CAD build for the part. Positions are in the model's coordinates, mm. A direction names the side the tool comes from. Give positions to 0.01 mm unless a question says otherwise; leave off trailing zeros. Loops run counter-clockwise (first coordinate to the right, second up) from the corner with the lowest first, then second, coordinate; pieces in that order, holes last. Notation, with made-up numbers: (26.25, 15.5) - (43.25, 15.5) arc R18 cw to (43.25, 35.5) - close; hole circle Ø4 at (-4, 28). An arc over 180 degrees is marked (long way). Return JSON: item names as keys, results as strings.
from build123d import *

# Parameters (mm, degrees)
F0_W     = 970
F0_H     = 1730
F1_DEPTH = 50
F3_DEPTH = 50


with BuildPart() as f1:
    # F0 (on Front) → F1 (new body)
    with BuildSketch(Plane.XZ):
        Polygon((1020, 0), (0, 0), (0, -1830), (1070, -1830), (1070, 0), align=None)
        with Locations((535, -915)):
            Rectangle(F0_W, F0_H, mode=Mode.SUBTRACT)
    extrude(amount=F1_DEPTH)

    # F2 (on Front) → F3 (join)
    with BuildSketch(Plane.XZ):
        Polygon((1041.897844, -1737.005164), (842.641968, -1388.040984), (78.297675, -49.416571), (49.824655, -49.968854), (47.816185, -96.869479), (155.709775, -285.827511), (861.881588, -1522.572309), (1007.799248, -1778.123299), (1039.504766, -1783.232212), align=None)
    extrude(amount=F3_DEPTH)


solid = f1.part
1. Cut at C-C, the plane x = 989. Write the cut outline in (y, z).
Values follow:
{"outline": "(-50, -1830) - (0, -1830) - (0, -1780) - (-50, -1780) - close; (-50, -1745.2) - (0, -1745.2) - (0, -1644.36) - (-50, -1644.36) - close; (-50, -50) - (0, -50) - (0, 0) - (-50, 0) - close"}
2. Cut at B-B, the plane z = -1079.5. Write the cut outline in (x, y).
Values follow:
{"outline": "(0, -50) - (50, -50) - (50, 0) - (0, 0) - close; (608.89, -50) - (666.47, -50) - (666.47, 0) - (608.89, 0) - close; (1020, -50) - (1070, -50) - (1070, 0) - (1020, 0) - close"}
3. Drill centre lines: probe 1 along Z at (x, y) = (428.5, -15); probe 2 along Z at (x, y) = (702.5, -30); probe 3 along X at (y, z) = (-20, -284). Where is each one in solid material? Low to high.
Values follow:
{"probe 1": "z = -1830 to -1780, -763.58 to -662.74, -50 to 0", "probe 2": "z = -1830 to -1780, -1243.44 to -1142.61, -50 to 0", "probe 3": "x = 0 to 50, 154.67 to 212.24, 1020 to 1070"}
4. Pull direction Z, two halves, no side cores. Call faces 1 (the face through (1020, -25, -886)), 2 (the face through (533, -50, -911)), 3 (the face through (542, -25, 0)): +Z half, -Z half, draft (parallel to the pull), parting line (faces both ways), or undercut.
Values follow:
{"face 1": "undercut", "face 2": "draft", "face 3": "+Z half"}
5. Which spindle directions (+Z, -Z, +X, -X, +Y, -Y) get a long thin tool onto all of the face, cutting with end or side? Do faces 4 (the face through (50, -25, -952)), 5 (the face through (533, 0, -911)). Say none if no direction does.
Values follow:
{"face 4": "+Y, -Y", "face 5": "+Z, -Z, +X, -X, +Y"}
6. Cut at A-A, the plane y = -38. Write the cut outline in (x, z), plus the area to 3 significant figures.
Values follow:
{"outline": "(0, -1830) - (1070, -1830) - (1070, 0) - (0, 0) - close; hole (50, -1780) - (1019.45, -1780) - (1007.8, -1778.12) - (50, -100.69) - close; hole (78.63, -50) - (1020, -1698.65) - (1020, -50) - close", "area": "377,000 mm²"}
